Build history of the part. All positions in model axes, mm. Face numbers are marked on the shaded views. A direction names the side the tool comes from. Give positions to 0.01 mm unless a question says otherwise; leave off trailing zeros. Write each loop counter-clockwise with the first axis right and the second up, starting at its lowest first coordinate (ties: lowest second). Pieces come first, ordered by that corner, then holes. Notation, with made-up numbers: (-15.5, -37.75) -> (-2.5, -37.75) arc R20 cw to (-2.5, -31.75) -> close; hole circle Ø11 at (60.25, 23). An arc over 180 degrees is marked (long way). Put each result on its own line as item: value. Start each with the question number.
Item 1: Flat gauge pins, fed straight in: pin 1 Ø2 at (x, z) = (-1.5, 3) entering from -Y; pin 2 Ø3 at (x, y) = (-12.5, -10.5) entering from -Z; pin 3 Ø5 at (x, y) = (0, -13) entering from +Z; pin 4 Ø2.5 at (x, y) = (13, 0) entering from -Z. Where does each tip first touch, or does it go through?
Item 2: Two-plate mould, pull along X, no slides. Class the marked faces 1, 2, 3 and 4: pulls with the +X half, pulls with the -X half, needs draft (parallel to the pull), parting line crosses it, or undercut.
Item 3: Slice it at C-C, the plane z = 1.35. List the corners of the cut face in (x, y).
Item 4: Drill centre lines: line 1 along Y through (x, z) = (0, 4.5); line 2 along Y through (x, z) = (0, 1.05); line 3 along X through (y, z) = (2, 3.1). Where is each one in solid material? Low to high.
Item 5: Slice it at D-D, the plane x = 13. List the corners of the cut face in (y, z).
Item 6: Tool access for the marked faces 5 and 6: list every direction of +Z, -Z, +X, -X, +Y, -Y with a clear straight run to the whole face (end or side of a thin tool).
Item 7: Slice it at A-A, the plane x = 0. List the corners of the cut face in (y, z).
Item 8: Slice it at B-B, the plane y = -13.5. List the corners of the cut face in (x, z), plus the area to 3 significant figures.
```python
from build123d import *

# Parameters (mm, degrees)
SKETCH1_R           = 21
SKETCH1_R_2         = 2.85
BOSS_EXTRUDE1_DEPTH = 6
SKETCH1_4_R         = 2.85
SKETCH1_4_R_2       = 1.6
BOSS_EXTRUDE2_DEPTH = 3


with BuildPart() as part:
    # Sketch1 → Boss-Extrude1 (new body)
    with BuildSketch(Plane(origin=(0, 0, 0), x_dir=(0, 1, 0), z_dir=(0, 0, 1))):
        with Locations(Location((0, 0, 0), (0, 0, 270))):
            Circle(SKETCH1_R)
        with Locations(Location((-13, 0, 0), (0, 0, 270))):
            Circle(SKETCH1_R_2, mode=Mode.SUBTRACT)
        with Locations(Location((0, -13, 0), (0, 0, 270))):
            Circle(SKETCH1_R_2, mode=Mode.SUBTRACT)
        with Locations(Location((13, 0, 0), (0, 0, 270))):
            Circle(SKETCH1_R_2, mode=Mode.SUBTRACT)
        with Locations(Location((0, 13, 0), (0, 0, 270))):
            Circle(SKETCH1_R_2, mode=Mode.SUBTRACT)
    extrude(amount=BOSS_EXTRUDE1_DEPTH)

    # Sketch1_4 → Boss-Extrude2 (add)
    # profile 1 of 4: a face of its own
    with BuildSketch(Plane(origin=(0, 0, 0), x_dir=(0, 1, 0), z_dir=(0, 0, 1))):
        with Locations(Location((-13, 0, 0), (0, 0, 270))):
            Circle(SKETCH1_4_R)
        with Locations(Location((-13, 0, 0), (0, 0, 270))):
            Circle(SKETCH1_4_R_2, mode=Mode.SUBTRACT)
    # profile 2 of 4: a face of its own
    with BuildSketch(Plane(origin=(0, 0, 0), x_dir=(0, 1, 0), z_dir=(0, 0, 1))):
        with Locations(Location((0, 13, 0), (0, 0, 270))):
            Circle(SKETCH1_4_R)
        with Locations(Location((0, 13, 0), (0, 0, 270))):
            Circle(SKETCH1_4_R_2, mode=Mode.SUBTRACT)
    # profile 3 of 4: a face of its own
    with BuildSketch(Plane(origin=(0, 0, 0), x_dir=(0, 1, 0), z_dir=(0, 0, 1))):
        with Locations(Location((13, 0, 0), (0, 0, 270))):
            Circle(SKETCH1_4_R)
        with Locations(Location((13, 0, 0), (0, 0, 270))):
            Circle(SKETCH1_4_R_2, mode=Mode.SUBTRACT)
    # profile 4 of 4: a face of its own
    with BuildSketch(Plane(origin=(0, 0, 0), x_dir=(0, 1, 0), z_dir=(0, 0, 1))):
        with Locations(Location((0, -13, 0), (0, 0, 270))):
            Circle(SKETCH1_4_R)
        with Locations(Location((0, -13, 0), (0, 0, 270))):
            Circle(SKETCH1_4_R_2, mode=Mode.SUBTRACT)
    extrude(amount=BOSS_EXTRUDE2_DEPTH)


solid = part.part
```
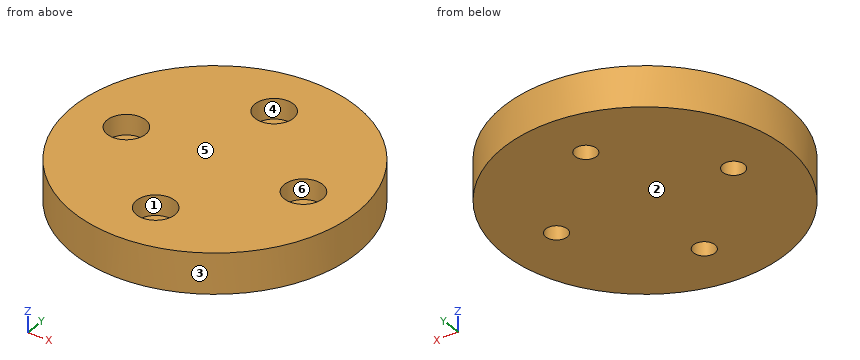
Values follow:
1. pin 1: y = -20.99
1. pin 2: z = 0
1. pin 3: z = 3
1. pin 4: through
2. face 1: undercut
2. face 2: needs draft
2. face 3: parting line crosses it
2. face 4: undercut
3. outline: circle Ø42 at (0, 0); hole circle Ø3.2 at (-13, 0); hole circle Ø3.2 at (0, -13); hole circle Ø3.2 at (0, 13); hole circle Ø3.2 at (13, 0)
4. line 1: -21 to -15.85, -10.15 to 10.15, 15.85 to 21
4. line 2: -21 to -14.6, -11.4 to 11.4, 14.6 to 21
4. line 3: -20.9 to -15.03, -10.97 to 10.97, 15.03 to 20.9
5. outline: (-16.49, 0) -> (-1.6, 0) -> (-1.6, 3) -> (-2.85, 3) -> (-2.85, 6) -> (-16.49, 6) -> close; (1.6, 0) -> (16.49, 0) -> (16.49, 6) -> (2.85, 6) -> (2.85, 3) -> (1.6, 3) -> close
6. face 5: +Z, +X, -X, +Y, -Y
6. face 6: +Z
7. outline: (-21, 0) -> (-14.6, 0) -> (-14.6, 3) -> (-15.85, 3) -> (-15.85, 6) -> (-21, 6) -> close; (-11.4, 0) -> (11.4, 0) -> (11.4, 3) -> (10.15, 3) -> (10.15, 6) -> (-10.15, 6) -> (-10.15, 3) -> (-11.4, 3) -> close; (14.6, 0) -> (21, 0) -> (21, 6) -> (15.85, 6) -> (15.85, 3) -> (14.6, 3) -> close
8. outline: (-16.09, 0) -> (-1.52, 0) -> (-1.52, 3) -> (-2.81, 3) -> (-2.81, 6) -> (-16.09, 6) -> close; (1.52, 0) -> (16.09, 0) -> (16.09, 6) -> (2.81, 6) -> (2.81, 3) -> (1.52, 3) -> close
8. area: 167 mm2
